Work out the finished part from the listing and answer in its coordinate system (mm). Round coordinates to 2 decimals unless told otherwise and drop trailing zeros. Loops run counter-clockwise (first coordinate to the right, second up) from the corner with the lowest first, then second, coordinate; pieces in that order, holes last.
```python
from build123d import *

# Parameters (mm, degrees)
BOSS_EXTRUDE1_DEPTH      = 2.3876
BOSS_EXTRUDE1_DEPTH_BACK = 2.3876
SKETCH4_R                = 3.2639
CUT_EXTRUDE1_DEPTH       = 5.7752


with BuildPart() as part:
    # Sketch3 → Boss-Extrude1 (new body, two sides)
    with BuildSketch(Plane.XY) as boss_extrude1_sk:
        Polygon((50.8, -25.4), (50.8, -50.8), (-50.8, -50.8), (-50.8, 50.8), (-25.4, 50.8), align=None)
    extrude(amount=BOSS_EXTRUDE1_DEPTH)
    extrude(boss_extrude1_sk.sketch, amount=-BOSS_EXTRUDE1_DEPTH_BACK)

    # Sketch4 → Cut-Extrude1 (cut, through all)
    with BuildSketch(Plane.XY.offset(2.3876)):
        with Locations((-38.1, -38.1)):
            Circle(SKETCH4_R)
        with Locations((-12.7, -38.1)):
            Circle(SKETCH4_R)
        with Locations((12.7, -38.1)):
            Circle(SKETCH4_R)
        with Locations((-38.1, -12.7)):
            Circle(SKETCH4_R)
        with Locations((-38.1, 12.7)):
            Circle(SKETCH4_R)
        with Locations((38.1, -38.1)):
            Circle(SKETCH4_R)
        with Locations((-38.1, 38.1)):
            Circle(SKETCH4_R)
    extrude(amount=-CUT_EXTRUDE1_DEPTH, mode=Mode.SUBTRACT)


solid = part.part
```
1. Consider probe 1 along Y at (x, z) = (-38.1, 0.2); probe 2 along X at (y, z) = (-39, -2.1). Determine where each line is inside the solid, lowest interval first.
Answer key:
probe 1: y = -50.8 to -41.36, -34.84 to -15.96, -9.44 to 9.44, 15.96 to 34.84, 41.36 to 50.8
probe 2: x = -50.8 to -41.24, -34.96 to -15.84, -9.56 to 9.56, 15.84 to 34.96, 41.24 to 50.8
2. Find section A-A (y = 12.7). Write down the section's boundary in (x, z).
Answer key:
outline: (-50.8, -2.39) - (-41.36, -2.39) - (-41.36, 2.39) - (-50.8, 2.39) - close; (-34.84, -2.39) - (12.7, -2.39) - (12.7, 2.39) - (-34.84, 2.39) - close
3. Find section C-C (y = -38.1). Write down the section's boundary in (x, z).
Answer key:
outline: (-50.8, -2.39) - (-41.36, -2.39) - (-41.36, 2.39) - (-50.8, 2.39) - close; (-34.84, -2.39) - (-15.96, -2.39) - (-15.96, 2.39) - (-34.84, 2.39) - close; (-9.44, -2.39) - (9.44, -2.39) - (9.44, 2.39) - (-9.44, 2.39) - close; (15.96, -2.39) - (34.84, -2.39) - (34.84, 2.39) - (15.96, 2.39) - close; (41.36, -2.39) - (50.8, -2.39) - (50.8, 2.39) - (41.36, 2.39) - close
4. Determine the mould class of faces 1 (the face through (-11, -11, -2.388)), 2 (the face through (12.2, 13.2, 0)), 3 (the face through (-50.8, -1, 0)), 4 (the face through (-40.69, -40.086, 0.033)) for opening direction X: +X half, -X half, draft (parallel to the pull), parting line (faces both ways), or undercut.
Answer key:
face 1: draft
face 2: +X half
face 3: -X half
face 4: undercut
